Model file for the job. Use its own axes, mm. A direction names the side the tool comes from. Give positions to 0.01 mm unless a question says otherwise; leave off trailing zeros. Loops run counter-clockwise (first coordinate to the right, second up) from the corner with the lowest first, then second, coordinate; pieces in that order, holes last. Notation, with made-up numbers: (9, 50.25) - (40, 50.25) arc R22 cw to (40, 67.25) - close; hole circle Ø3 at (47, -38). An arc over 180 degrees is marked (long way). Use a Markdown table: item, result.
from build123d import *

# Parameters (mm, degrees)
SKETCH2_W               = 121
SKETCH2_H               = 171
BOSS_EXTRUDE1_DEPTH     = 88
SKETCH4_W               = 115
SKETCH4_H               = 165
CUT_EXTRUDE1_DEPTH      = 82
SKETCH5_W               = 41
SKETCH5_H               = 121.6
CUT_EXTRUDE2_DEPTH      = 3.2
SKETCH6_W               = 69.6
SKETCH6_H               = 9
BOSS_EXTRUDE2_DEPTH     = 2.5
SKETCH7_W               = 19.4
SKETCH7_H               = 68.6
CUT_EXTRUDE3_DEPTH      = 3.4
SKETCH9_W               = 70.2
SKETCH9_H               = 66.6
CUT_EXTRUDE4_DEPTH      = 3.4
SKETCH10_W              = 65.5
SKETCH10_H              = 57.2
CUT_EXTRUDE5_DEPTH      = 2.6
SKETCH11_R              = 10.5
SKETCH11_R_2            = 10
CUT_EXTRUDE6_DEPTH      = 228.213555934
BOSS_EXTRUDE4_DEPTH     = 7.5
BOSS_EXTRUDE5_DEPTH     = 9
CUT_EXTRUDE10_DEPTH     = 2
BOSS_EXTRUDE6_DEPTH     = 72.5
SKETCH18_R              = 2
CUT_EXTRUDE11_DEPTH     = 5
SKETCH19_R              = 2
CUT_EXTRUDE12_DEPTH     = 5
SKETCH20_R              = 4.75
BOSS_EXTRUDE7_DEPTH     = 5
SKETCH21_R              = 2
CUT_EXTRUDE13_DEPTH     = 5
SKETCH22_R              = 2.5
CUT_EXTRUDE14_DEPTH     = 6
BOSS_EXTRUDE17_REACH    = 229.214
BOSS_EXTRUDE18_REACH    = 229.214
BOSS_EXTRUDE19_DEPTH    = 5
BOSS_EXTRUDE20_DEPTH    = 20
BOSS_EXTRUDE22_DEPTH    = 20
CHAMFER1_SIZE           = 10
CHAMFER2_SIZE           = 10
SKETCH38_R              = 2.5
CUT_EXTRUDE15_DEPTH     = 5
CHAMFER3_SIZE           = 5
CUT_EXTRUDE16_START     = -3
CUT_EXTRUDE16_OUTLINE_R = 10.5
CUT_EXTRUDE16_DEPTH     = 3
CUT_EXTRUDE17_DEPTH     = 1
SKETCH42_W              = 17
SKETCH42_H              = 88
CUT_EXTRUDE18_DEPTH     = 1
SKETCH44_W              = 77.75
SKETCH44_H              = 20
BOSS_EXTRUDE25_DEPTH    = 1
BOSS_EXTRUDE26_DEPTH    = 2.6
SKETCH46_R              = 1.5
CUT_EXTRUDE19_DEPTH     = 2.6
FILLET1_R               = 1
SKETCH48_W              = 25
SKETCH48_H              = 20
CUT_EXTRUDE21_DEPTH     = 10
BOSS_EXTRUDE27_DEPTH    = 2
SKETCH50_R              = 2
CUT_EXTRUDE22_DEPTH     = 5


# Read off the part's stored shape, not the designer's step: Cut-Extrude16
with BuildPart() as part:
    # Sketch2 → Boss-Extrude1 (new body)
    with BuildSketch(Plane(origin=(0, 0, 0), x_dir=(1, 0, 0), z_dir=(0, 1, 0))):
        with Locations((60.5, 85.5)):
            Rectangle(SKETCH2_W, SKETCH2_H)
    extrude(amount=BOSS_EXTRUDE1_DEPTH)

    # Sketch4 → Cut-Extrude1 (cut)
    with BuildSketch(Plane(origin=(0, 88, 0), x_dir=(1, 0, 0), z_dir=(0, 1, 0))):
        with Locations((57.5, 82.5)):
            Rectangle(SKETCH4_W, SKETCH4_H)
    extrude(amount=-CUT_EXTRUDE1_DEPTH, mode=Mode.SUBTRACT)

    # Sketch5 → Cut-Extrude2 (cut)
    with BuildSketch(Plane.XZ):
        with Locations((20.5, -85.5)):
            Rectangle(SKETCH5_W, SKETCH5_H)
    extrude(amount=-CUT_EXTRUDE2_DEPTH, mode=Mode.SUBTRACT)

    # Sketch6 → Boss-Extrude2 (add)
    with BuildSketch(Plane.XZ):
        with Locations((60.5, 4.5)):
            Rectangle(SKETCH6_W, SKETCH6_H)
    extrude(amount=-BOSS_EXTRUDE2_DEPTH)

    # Sketch7 → Cut-Extrude3 (cut)
    with BuildSketch(Plane(origin=(121, 0, 0), x_dir=(0, 0, -1), z_dir=(1, 0, 0))):
        with Locations((9.7, 44)):
            Rectangle(SKETCH7_W, SKETCH7_H)
    extrude(amount=-CUT_EXTRUDE3_DEPTH, mode=Mode.SUBTRACT)

    # Sketch9 → Cut-Extrude4 (cut)
    with BuildSketch(Plane(origin=(0, 0, -171), x_dir=(-1, 0, 0), z_dir=(0, 0, -1))):
        with Locations((-35.1, 44)):
            Rectangle(SKETCH9_W, SKETCH9_H)
    extrude(amount=-CUT_EXTRUDE4_DEPTH, mode=Mode.SUBTRACT)

    # Sketch10 → Cut-Extrude5 (cut)
    with BuildSketch(Plane(origin=(0, 0, -167.6), x_dir=(-1, 0, 0), z_dir=(0, 0, -1))):
        with Locations((-32.75, 44)):
            Rectangle(SKETCH10_W, SKETCH10_H)
    extrude(amount=-CUT_EXTRUDE5_DEPTH, mode=Mode.SUBTRACT)

    # Sketch11 → Cut-Extrude6 (cut, through all)
    with BuildSketch(Plane(origin=(121, 0, 0), x_dir=(0, 0, -1), z_dir=(1, 0, 0))):
        with Locations((136.5, 61)):
            Circle(SKETCH11_R)
        with Locations((96.5, 61)):
            Circle(SKETCH11_R)
        with Locations((42.4, 50)):
            Circle(SKETCH11_R_2)
    extrude(amount=-CUT_EXTRUDE6_DEPTH, mode=Mode.SUBTRACT)

    # Sketch14 → Boss-Extrude4 (add)
    with BuildSketch(Plane(origin=(0, 86, 0), x_dir=(1, 0, 0), z_dir=(0, 1, 0))):
        Polygon((115, 142.372583002), (115, 165), (92.372583002, 165), align=None)
    extrude(amount=-BOSS_EXTRUDE4_DEPTH)

    # Sketch15 → Boss-Extrude5 (add)
    with BuildSketch(Plane(origin=(0, 88, 0), x_dir=(1, 0, 0), z_dir=(0, 1, 0))):
        Polygon((115, 105), (115, 82.372583002), (92.372583002, 105), (115, 127.627416998), align=None)
    extrude(amount=-BOSS_EXTRUDE5_DEPTH)

    # Sketch16 → Cut-Extrude10 (cut)
    with BuildSketch(Plane(origin=(0, 88, 0), x_dir=(1, 0, 0), z_dir=(0, 1, 0))):
        Polygon((115, 127.627416998), (115, 105), (92.372583002, 105), align=None)
    extrude(amount=-CUT_EXTRUDE10_DEPTH, mode=Mode.SUBTRACT)

    # Sketch17 → Boss-Extrude6 (add)
    with BuildSketch(Plane(origin=(0, 6, 0), x_dir=(1, 0, 0), z_dir=(0, 1, 0))):
        Polygon((115, 165), (108, 165), (115, 158), align=None)
    extrude(amount=BOSS_EXTRUDE6_DEPTH)

    # Sketch18 → Cut-Extrude11 (cut)
    with BuildSketch(Plane(origin=(0, 86, 0), x_dir=(1, 0, 0), z_dir=(0, 1, 0))):
        with Locations(Location((109.343145751, 159.343145751, 0), (0, 0, 270))):
            Circle(SKETCH18_R)
        with Locations(Location((109.343145751, 110.656854249, 0), (0, 0, 270))):
            Circle(SKETCH18_R)
    extrude(amount=-CUT_EXTRUDE11_DEPTH, mode=Mode.SUBTRACT)

    # Sketch19 → Cut-Extrude12 (cut)
    with BuildSketch(Plane(origin=(0, 88, 0), x_dir=(1, 0, 0), z_dir=(0, 1, 0))):
        with Locations(Location((109.343145751, 99.343145751, 0), (0, 0, 270))):
            Circle(SKETCH19_R)
    extrude(amount=-CUT_EXTRUDE12_DEPTH, mode=Mode.SUBTRACT)

    # Sketch20 → Boss-Extrude7 (add)
    with BuildSketch(Plane(origin=(0, 6, 0), x_dir=(1, 0, 0), z_dir=(0, 1, 0))):
        with Locations(Location((85, 47.7, 0), (0, 0, 90))):
            Circle(SKETCH20_R)
        with BuildLine():
            Line((27.85, 78.78), (88, 78.78))
            ThreePointArc((88, 78.78), (94, 84.78), (88, 90.78))
            Line((88, 90.78), (27.85, 90.78))
            ThreePointArc((27.85, 90.78), (21.85, 84.78), (27.85, 78.78))
        make_face()
    extrude(amount=BOSS_EXTRUDE7_DEPTH)

    # Sketch21 → Cut-Extrude13 (cut)
    with BuildSketch(Plane(origin=(0, 11, 0), x_dir=(1, 0, 0), z_dir=(0, 1, 0))):
        with Locations(Location((85, 47.7, 0), (0, 0, 270))):
            Circle(SKETCH21_R)
    extrude(amount=-CUT_EXTRUDE13_DEPTH, mode=Mode.SUBTRACT)

    # Sketch22 → Cut-Extrude14 (cut)
    with BuildSketch(Plane(origin=(0, 11, 0), x_dir=(1, 0, 0), z_dir=(0, 1, 0))):
        with Locations(Location((88, 84.78, 0), (0, 0, 270))):
            Circle(SKETCH22_R)
        with Locations(Location((27.85, 84.78, 0), (0, 0, 270))):
            Circle(SKETCH22_R)
    extrude(amount=-CUT_EXTRUDE14_DEPTH, mode=Mode.SUBTRACT)

    # Boss-Extrude17: up to this plane
    boss_extrude17_end = Plane(origin=(108, 88.399494937, -165), z_dir=(0.7071067811865476, 0, -0.7071067811865476))
    # Sketch33 → Boss-Extrude17 (add, up to the surface)
    with BuildSketch(Plane.XY, mode=Mode.PRIVATE) as boss_extrude17_sk1:
        Polygon((108, 6), (115, 13), (115, 6), align=None)
    boss_extrude17_tool1 = split(extrude(boss_extrude17_sk1.sketch, amount=-BOSS_EXTRUDE17_REACH, mode=Mode.PRIVATE), bisect_by=boss_extrude17_end, keep=Keep.BOTH, mode=Mode.PRIVATE)
    add(boss_extrude17_tool1.solids().sort_by_distance((112.666667, 8.333333, 0))[0])

    # Boss-Extrude18: up to this plane
    boss_extrude18_end = Plane(origin=(108, 88.399494937, -165), z_dir=(0.7071067811865476, 0, -0.7071067811865476))
    # Sketch34 → Boss-Extrude18 (add, up to the surface)
    with BuildSketch(Plane.ZY, mode=Mode.PRIVATE) as boss_extrude18_sk1:
        Polygon((-165, 6), (-165, 13), (-158, 6), align=None)
    boss_extrude18_tool1 = split(extrude(boss_extrude18_sk1.sketch, amount=-BOSS_EXTRUDE18_REACH, mode=Mode.PRIVATE), bisect_by=boss_extrude18_end, keep=Keep.BOTH, mode=Mode.PRIVATE)
    add(boss_extrude18_tool1.solids().sort_by_distance((0, 8.333333, -162.666667))[0])

    # Sketch35 → Boss-Extrude19 (add)
    with BuildSketch(Plane(origin=(0, 6, 0), x_dir=(1, 0, 0), z_dir=(0, 1, 0))):
        with BuildLine():
            Line((82.006660465, 85.062632648), (80.255272868, 47.923750847))
            ThreePointArc((80.255272868, 47.923750847), (85.383052558, 52.434529622), (89.718985156, 47.158078331))
            Line((89.718985156, 47.158078331), (93.960823355, 84.095467366))
            ThreePointArc((93.960823355, 84.095467366), (87.516144137, 78.799541531), (82.006660465, 85.062632648))
        make_face()
    extrude(amount=BOSS_EXTRUDE19_DEPTH)

    # Sketch36 → Boss-Extrude20 (add)
    with BuildSketch(Plane(origin=(0, 6, 0), x_dir=(1, 0, 0), z_dir=(0, 1, 0))):
        Polygon((80.75, 128), (0, 128), (0, 125), (77.75, 125), (77.75, 121.6), (0, 121.6), (0, 117.6), (80.75, 117.6), align=None)
    extrude(amount=BOSS_EXTRUDE20_DEPTH)

    # Sketch37 → Boss-Extrude22 (add)
    with BuildSketch(Plane.XY.offset(-117.6)):
        Polygon((55.24, 26), (10.24, 26), (10.24, 6), (20.24, 6), (20.24, 21), (45.24, 21), (45.24, 6), (55.24, 6), align=None)
    extrude(amount=BOSS_EXTRUDE22_DEPTH)

    # Chamfer1
    chamfer1_edges = [part.edges().sort_by_distance(p)[0] for p in [
        (10.24, 6, -107.6),
    ]]
    chamfer(chamfer1_edges, length=CHAMFER1_SIZE)

    # Chamfer2
    chamfer2_edges = [part.edges().sort_by_distance(p)[0] for p in [
        (55.24, 6, -107.6),
    ]]
    chamfer(chamfer2_edges, length=CHAMFER2_SIZE)

    # Sketch38 → Cut-Extrude15 (cut)
    with BuildSketch(Plane(origin=(0, 26, 0), x_dir=(1, 0, 0), z_dir=(0, 1, 0))):
        with Locations(Location((32.74, 107.6, 0), (0, 0, 270))):
            Circle(SKETCH38_R)
    extrude(amount=-CUT_EXTRUDE15_DEPTH, mode=Mode.SUBTRACT)

    # Chamfer3
    chamfer3_edges = [part.edges().sort_by_distance(p)[0] for p in [
        (40.375, 6, -128),
    ]]
    chamfer(chamfer3_edges, length=CHAMFER3_SIZE)

    # Cut-Extrude16 outline → Cut-Extrude16 (cut)
    with BuildSketch(Plane.ZY.offset(-115).offset(CUT_EXTRUDE16_START)):
        with BuildLine():
            Line((-96.5, 78.5), (-136.5, 78.5))
            ThreePointArc((-136.5, 78.5), (-154, 61), (-136.5, 43.5))
            Line((-136.5, 43.5), (-96.5, 43.5))
            ThreePointArc((-96.5, 43.5), (-79, 61), (-96.5, 78.5))
        make_face()
        with Locations((-136.5, 61)):
            Circle(CUT_EXTRUDE16_OUTLINE_R, mode=Mode.SUBTRACT)
        with Locations((-96.5, 61)):
            Circle(CUT_EXTRUDE16_OUTLINE_R, mode=Mode.SUBTRACT)
    extrude(amount=CUT_EXTRUDE16_DEPTH, mode=Mode.SUBTRACT)

    # Sketch40 → Cut-Extrude17 (cut)
    with BuildSketch(Plane(origin=(0, 88, 0), x_dir=(1, 0, 0), z_dir=(0, 1, 0))):
        Polygon((117.1, 0), (118.9, 0), (118.9, 168.9), (0, 168.9), (0, 167.1), (117.1, 167.1), align=None)
    extrude(amount=-CUT_EXTRUDE17_DEPTH, mode=Mode.SUBTRACT)

    # Sketch42 → Cut-Extrude18 (cut)
    with BuildSketch(Plane(origin=(121, 0, 0), x_dir=(0, 0, -1), z_dir=(1, 0, 0))):
        with Locations((159.5, 44)):
            Rectangle(SKETCH42_W, SKETCH42_H)
    extrude(amount=-CUT_EXTRUDE18_DEPTH, mode=Mode.SUBTRACT)

    # Sketch44 → Boss-Extrude25 (add)
    with BuildSketch(Plane.XY.offset(-125)):
        with Locations((38.875, 16)):
            Rectangle(SKETCH44_W, SKETCH44_H)
    extrude(amount=BOSS_EXTRUDE25_DEPTH)

    # Sketch45 → Boss-Extrude26 (add)
    with BuildSketch(Plane(origin=(0, 0, -167.6), x_dir=(-1, 0, 0), z_dir=(0, 0, -1))):
        Polygon((-65.5, 72.6), (-65.5, 62.6), (-55.5, 72.6), align=None)
        Polygon((-65.5, 15.4), (-65.5, 25.4), (-55.5, 15.4), align=None)
    extrude(amount=-BOSS_EXTRUDE26_DEPTH)

    # Sketch46 → Cut-Extrude19 (cut)
    with BuildSketch(Plane(origin=(0, 0, -167.6), x_dir=(-1, 0, 0), z_dir=(0, 0, -1))):
        with Locations((-62.3, 18.6)):
            Circle(SKETCH46_R)
        with Locations((-62.3, 69.8)):
            Circle(SKETCH46_R)
    extrude(amount=-CUT_EXTRUDE19_DEPTH, mode=Mode.SUBTRACT)

    # Fillet1
    fillet1_edges = [part.edges().sort_by_distance(p)[0] for p in [
        (117.1, 87.5, -167.1),
        (118.9, 87.5, -168.9),
    ]]
    fillet(fillet1_edges, radius=FILLET1_R)

    # Sketch48 → Cut-Extrude21 (cut)
    with BuildSketch(Plane(origin=(0, 6, 0), x_dir=(1, 0, 0), z_dir=(0, 1, 0))):
        with Locations((32.74, 107.6)):
            Rectangle(SKETCH48_W, SKETCH48_H)
    extrude(amount=-CUT_EXTRUDE21_DEPTH, mode=Mode.SUBTRACT)

    # Sketch49 → Boss-Extrude27 (add)
    with BuildSketch(Plane.XY.offset(-97.6)):
        Polygon((10.24, 16), (0.24, 6), (20.24, 6), (45.24, 6), (65.24, 6), (55.24, 16), (55.24, 26), (10.24, 26), align=None)
    extrude(amount=BOSS_EXTRUDE27_DEPTH)

    # Sketch50 → Cut-Extrude22 (cut)
    with BuildSketch(Plane.XZ):
        with Locations(Location((105, -159.5, 0), (0, 0, 270))):
            Circle(SKETCH50_R)
    extrude(amount=-CUT_EXTRUDE22_DEPTH, mode=Mode.SUBTRACT)


solid = part.part
(1) Mould opens along X. For faces 5 (the flat face through (66, 44, -167.6)), 6 (the flat face through (0, 82, -168)), 7 (the cylindrical face through (106.352, 2.465, -158.026)) say: pulls with the +X half, pulls with the -X half, needs draft (parallel to the pull), parting line crosses it, or undercut.
Computed:
| item | result |
|---|---|
| face 5 | needs draft |
| face 6 | pulls with the -X half |
| face 7 | undercut |
(2) Slice it at D-D, the plane x = 105. Write the cut outline in (y, z), plus the area to 3 significant figures.
Computed:
| item | result |
|---|---|
| outline | (0, -171) - (88, -171) - (88, -168.9) - (87, -168.9) - (87, -167.1) - (88, -167.1) - (88, -165) - (86, -165) - (86, -152.37) - (78.5, -152.37) - (78.5, -165) - (13, -165) - (6, -158) - (6, 0) - (0, 0) - (0, -157.5) - (5, -157.5) - (5, -161.5) - (0, -161.5) - close; (79, -117.63) - (86, -117.63) - (86, -105) - (88, -105) - (88, -92.37) - (79, -92.37) - close |
| area | 1,820 mm² |
(3) Slice it at B-B, the plane z = -14.5. Write the cut outline in (x, y).
Computed:
| item | result |
|---|---|
| outline | (0, 0) - (121, 0) - (121, 9.7) - (117.6, 9.7) - (117.6, 78.3) - (121, 78.3) - (121, 88) - (118.9, 88) - (118.9, 87) - (117.1, 87) - (117.1, 88) - (115, 88) - (115, 13) - (108, 6) - (0, 6) - close |
(4) Pin check, flat tips, straight feed: P1, Ø8, axis at x = 86, y = 57, coming from the +Z side; P2, Ø5, axis at x = 62.3, y = 18.6, coming from the -Z side; P3, Ø16, axis at x = 33.5, z = -111.5, coming from the -Y side. Stop position of each tip, or through.
Computed:
| item | result |
|---|---|
| P1 | z = -165 |
| P2 | z = -167.6 |
| P3 | y = 3.2 |
(5) Drill centre lines: probe 1 along Z at (x, y) = (38, 17); probe 2 along Z at (x, y) = (71, 17); probe 3 along Z at (x, y) = (43.5, 22.5). Where is each one in solid material? Low to high. Write a range as [from, to].
Computed:
| item | result |
|---|---|
| probe 1 | [-128, -124], [-121.6, -117.6], [-97.6, -95.6] |
| probe 2 | [-171, -165], [-128, -124], [-121.6, -117.6] |
| probe 3 | [-128, -124], [-121.6, -95.6] |
(6) 3-axis set-ups, long thin cutter, end or side, ignore diameter. For faces 1 (the flat face through (55.24, 21, -107)), 2 (the flat face through (5.31, 11.07, -106.75)), 3 (the flat face through (32, 16, -95.6)), 4 (the flat face through (80.75, 16, -123)): which of +Z, -Z, +X, -X, +Y, -Y reach the whole face in a straight line?
Computed:
| item | result |
|---|---|
| face 1 | +Z, +Y |
| face 2 | +Z, -X, +Y |
| face 3 | -X, +Y |
| face 4 | +Y |
